Geometry: final body of the model. Coordinates: model frame, mm. Face numbers are marked on the shaded views. Give positions to 0.01 mm unless a question says otherwise; leave off trailing zeros. Write each loop counter-clockwise with the first axis right and the second up, starting at its lowest first coordinate (ties: lowest second). Pieces come first, ordered by that corner, then holes. Notation, with made-up numbers: M 44.25,4 L 101.25,4 A10 ccw 101.25,8 Z; hole C 82,-18 d4. An arc over 180 degrees is marked long. Use one line per item in the form item = value. Start each with the question number.
Item 1: Section query C-C on z = 33. Return loops of the section in (x, y), then the cut area to 3 significant figures.
Item 2: Section query A-A on z = 0. Return loops of the section in (x, y).
Item 3: Section query B-B on x = 0. Return loops of the section in (y, z), then the cut area to 3 significant figures.
Item 4: Material intervals for line 1 along Z through (x, y) = (-2.5, -7); line 2 along X through (y, z) = (-5.5, 0.5); line 3 along X through (y, z) = (-8.5, 1.5), sorted ascending. Write a range as from..to.
Item 5: Section query D-D on y = -2.5. Give the number of separate pieces and of enclosed holes in the cut face, then the cut area to 3 significant figures.
Item 6: Contact query for flat-ended pins moving along their axis: P1, Ø12, axis at y = -30.5, z = -6, coming from the -X side; P2, Ø6, axis at x = 0, z = -31.41, coming from the -Y side; P3, Ø12, axis at y = -8, z = 28.5, coming from the +X side; P4, Ø13, axis at x = 22.21, z = 22.21, coming from the -Y side. Output: stop coordinate, or through.
Item 7: Pull-direction query (X, two-part tool) for the marked faces 1, 2 and 3; classes: released by +X, released by -X, zero draft, split by the parting line, or undercut.
from build123d import *

# Parameters (mm, degrees)
F0_R      = 40
F1_DEPTH  = 10
F2_R      = 22.604582
F2_R_2    = 16.387311
F3_DEPTH  = 25
F3_FACE_R = 16.387311
F4_DEPTH  = 25
F5_R      = 5
F6_DEPTH  = 25


with BuildPart() as f1:
    # F0 (on Front) → F1 (new body)
    with BuildSketch(Plane.XZ):
        Circle(F0_R)
    extrude(amount=F1_DEPTH)

    # F2 (on face) → F3 (join)
    with BuildSketch(Plane.XZ.offset(10)):
        Circle(F2_R)
        Circle(F2_R_2, mode=Mode.SUBTRACT)
    extrude(amount=F3_DEPTH)

    # F3_face (on face) → F4 (cut)
    with BuildSketch(Plane.XZ.offset(10)):
        Circle(F3_FACE_R)
    extrude(amount=-F4_DEPTH, mode=Mode.SUBTRACT)

    # F5 (on face) → F6 (cut)
    with BuildSketch(Plane.XZ.offset(10)):
        with Locations((0, 31.406611)):
            Circle(F5_R)
        with Locations((-22.207828, 22.207828)):
            Circle(F5_R)
        with Locations((-31.406611, 0)):
            Circle(F5_R)
        with Locations((-22.207828, -22.207828)):
            Circle(F5_R)
        with Locations((0, -31.406611)):
            Circle(F5_R)
        with Locations((22.207828, -22.207828)):
            Circle(F5_R)
        with Locations((31.406611, 0)):
            Circle(F5_R)
        with Locations((22.207828, 22.207828)):
            Circle(F5_R)
    extrude(amount=-F6_DEPTH, mode=Mode.SUBTRACT)


solid = f1.part
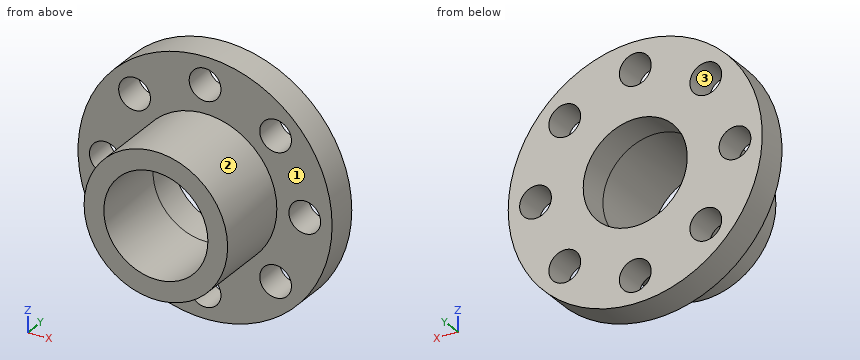
Answer sheet:
q1.outline = M -22.61,-10 L -4.74,-10 L -4.74,0 L -22.61,0 Z; M 4.74,-10 L 22.61,-10 L 22.61,0 L 4.74,0 Z
q1.area = 357 mm2
q2.outline = M -40,-10 L -36.41,-10 L -36.41,0 L -40,0 Z; M -26.41,-10 L -22.6,-10 L -22.6,-35 L -16.39,-35 L -16.39,0 L -26.41,0 Z; M 16.39,-35 L 22.6,-35 L 22.6,-10 L 26.41,-10 L 26.41,0 L 16.39,0 Z; M 36.41,-10 L 40,-10 L 40,0 L 36.41,0 Z
q3.outline = M -35,-22.6 L -10,-22.6 L -10,-26.41 L 0,-26.41 L 0,-16.39 L -35,-16.39 Z; M -35,16.39 L 0,16.39 L 0,26.41 L -10,26.41 L -10,22.6 L -35,22.6 Z; M -10,-40 L 0,-40 L 0,-36.41 L -10,-36.41 Z; M -10,36.41 L 0,36.41 L 0,40 L -10,40 Z
q3.area = 583 mm2
q4.line_1 = -39.92..-35.74, -27.08..-16.2, 16.2..27.08, 35.74..39.92
q4.line_2 = -40..-36.38, -26.43..-16.38, 16.38..26.43, 36.38..40
q4.line_3 = -39.97..-36.18, -26.64..-16.32, 16.32..26.64, 36.18..39.97
q5.separate_pieces = 1
q5.enclosed_holes = 9
q5.area = 3,550 mm2
q6.P1 = -22.6
q6.P2 = through
q6.P3 = 33.07
q6.P4 = -10
q7.face_1 = zero draft
q7.face_2 = split by the parting line
q7.face_3 = undercut
